Verification items for the finished model (mm, model axes). Coordinates: 2 decimals unless noted, no trailing zeros.
Q1. Cross-section at A-A, the plane y = 200.5. Count the separate pieces of the cut face and the enclosed holes in it, and give its area (3 significant figures).
Q2. Thickness scan on line 1 (X direction, y = 241.5, z = -19); line 2 (Y direction, x = -141.5, z = -15); line 3 (Z direction, x = -145, y = 227). Record the ranges inside material, lowest first.
Q3. Depth check by flat-ended pin: P1, Ø10, axis at x = -122, y = 217.5, coming from the +Z side; P2, Ø1, axis at y = 237.5, z = -21.5, coming from the +X side; P3, Ø3, axis at x = -133, y = 226.5, coming from the -Z side. Enter the tip coordinate at first touch or a pass-through.
from build123d import *

# Parameters (mm, degrees)
SKETCH1_R           = 11.43
BOSS_EXTRUDE1_DEPTH = 2.54
SKETCH2_R           = 9.9949
BOSS_EXTRUDE2_DEPTH = 50.8
SKETCH3_R           = 5.715
BOSS_EXTRUDE3_DEPTH = 1.016
SKETCH4_R           = 6.35
BOSS_EXTRUDE4_DEPTH = 21.336
SKETCH5_R           = 3.175
CUT_EXTRUDE1_DEPTH  = 99.13815411
SKETCH6_R           = 7.9375
CUT_EXTRUDE2_DEPTH  = 38.1


with BuildPart() as part:
    # Sketch1 → Boss-Extrude1 (new body)
    with BuildSketch(Plane(origin=(-129.203450499, 253.122013832, -50.271342949), x_dir=(0.8839119577418659, 0.40461078724322996, -0.23449895907520743), z_dir=(-0.4476862825736014, 0.8770605813697528, -0.1741887740435096))):
        with Locations(Location((-31.085661697, -28.519102589, 0), (0, 0, 166.223237714))):
            Circle(SKETCH1_R)
    extrude(amount=BOSS_EXTRUDE1_DEPTH)

    # Sketch2 → Boss-Extrude2 (add)
    with BuildSketch(Plane(origin=(-129.203450499, 253.122013832, -50.271342949), x_dir=(-0.8839119577418658, -0.4046107872432301, 0.23449895907520704), z_dir=(0.44768628257360144, -0.8770605813697528, 0.17418877404350955))):
        with Locations(Location((31.085661697, -28.519102589, 0), (0, 0, 13.776762286))):
            Circle(SKETCH2_R)
    extrude(amount=BOSS_EXTRUDE2_DEPTH)

    # Sketch3 → Boss-Extrude3 (add)
    with BuildSketch(Plane(origin=(-106.460987345, 208.567336298, -41.422553227), x_dir=(-0.8839119577418658, -0.40461078724323, 0.2344989590752073), z_dir=(0.44768628257360144, -0.8770605813697528, 0.17418877404350946))):
        with Locations(Location((31.085661697, -28.519102589, 0), (0, 0, 193.776762286))):
            Circle(SKETCH3_R)
    extrude(amount=BOSS_EXTRUDE3_DEPTH)

    # Sketch4 → Boss-Extrude4 (add)
    with BuildSketch(Plane(origin=(-106.006138081, 207.676242747, -41.245577433), x_dir=(-0.8839119577418657, -0.40461078724322985, 0.23449895907520799), z_dir=(0.4476862825736014, -0.8770605813697527, 0.1741887740435095))):
        with Locations(Location((31.085661697, -28.519102589, 0), (0, 0, 193.776762286))):
            Circle(SKETCH4_R)
    extrude(amount=BOSS_EXTRUDE4_DEPTH)

    # Sketch5 → Cut-Extrude1 (cut, through all)
    with BuildSketch(Plane(origin=(-130.340573657, 255.349747708, -50.713782435), x_dir=(0.8839119577418658, 0.40461078724323, -0.2344989590752073), z_dir=(-0.4476862825736014, 0.8770605813697528, -0.1741887740435095))):
        with Locations(Location((-31.085661697, -28.519102589, 0), (0, 0, 166.223237714))):
            Circle(SKETCH5_R)
    extrude(amount=-CUT_EXTRUDE1_DEPTH, mode=Mode.SUBTRACT)

    # Sketch6 → Cut-Extrude2 (cut)
    with BuildSketch(Plane(origin=(-130.340573657, 255.349747708, -50.713782435), x_dir=(0.8839119577418658, 0.40461078724323, -0.2344989590752073), z_dir=(-0.4476862825736014, 0.8770605813697528, -0.1741887740435095))):
        with Locations(Location((-31.085661697, -28.519102589, 0), (0, 0, 166.223237714))):
            Circle(SKETCH6_R)
    extrude(amount=-CUT_EXTRUDE2_DEPTH, mode=Mode.SUBTRACT)


solid = part.part
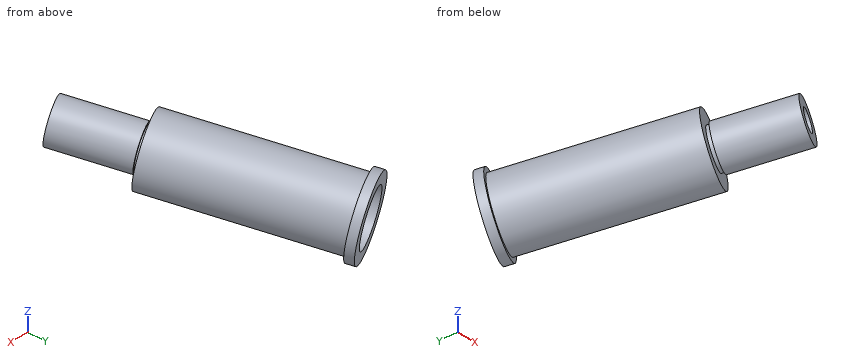
Check values:
1. separate pieces: 2
1. enclosed holes: 1
1. area: 152 mm2
2. line 1: x = -159.98 to -157.31, -142.66 to -140
2. line 2: y = 208.66 to 213.31, 243.08 to 247.72
2. line 3: z = -21.6 to -19.41, -4.14 to -1.96
3. P1: stops at z = -3.25
3. P2: stops at x = -140.48
3. P3: stops at z = -18.55
